```python
from build123d import *

# Parameters (mm, degrees)
CUT_EXTRUDE1_REACH = 6
SKETCH3_R          = 1.5875


with BuildPart() as part:
    # Sketch2 → Revolve1 (revolve)
    with BuildSketch(Plane.XY):
        Polygon((-16, -4), (0, -4), (0, -16.000000004), (-4, -16.000000004), (-4, -8), (-16, -8), align=None)
    revolve(axis=Axis((-12.310421286, 0, 0), (1, 0, 0)))

    # Sketch3 → Cut-Extrude1 (cut, up to next)
    with BuildSketch(Plane.ZY.offset(4), mode=Mode.PRIVATE) as cut_extrude1_sk1:
        with Locations((-9.525, 9.525)):
            Circle(SKETCH3_R)
    cut_extrude1_tool1 = extrude(cut_extrude1_sk1.sketch, amount=-CUT_EXTRUDE1_REACH, mode=Mode.PRIVATE) & part.part
    add(cut_extrude1_tool1.solids().sort_by_distance((-4, 9.525, -9.525))[0], mode=Mode.SUBTRACT)
    # Sketch3 → Cut-Extrude1 (cut, up to next)
    with BuildSketch(Plane.ZY.offset(4), mode=Mode.PRIVATE) as cut_extrude1_sk2:
        with Locations((-9.525, -9.525)):
            Circle(SKETCH3_R)
    cut_extrude1_tool2 = extrude(cut_extrude1_sk2.sketch, amount=-CUT_EXTRUDE1_REACH, mode=Mode.PRIVATE) & part.part
    add(cut_extrude1_tool2.solids().sort_by_distance((-4, -9.525, -9.525))[0], mode=Mode.SUBTRACT)
    # Sketch3 → Cut-Extrude1 (cut, up to next)
    with BuildSketch(Plane.ZY.offset(4), mode=Mode.PRIVATE) as cut_extrude1_sk3:
        with Locations((9.525, -9.525)):
            Circle(SKETCH3_R)
    cut_extrude1_tool3 = extrude(cut_extrude1_sk3.sketch, amount=-CUT_EXTRUDE1_REACH, mode=Mode.PRIVATE) & part.part
    add(cut_extrude1_tool3.solids().sort_by_distance((-4, -9.525, 9.525))[0], mode=Mode.SUBTRACT)
    # Sketch3 → Cut-Extrude1 (cut, up to next)
    with BuildSketch(Plane.ZY.offset(4), mode=Mode.PRIVATE) as cut_extrude1_sk4:
        with Locations((9.525, 9.525)):
            Circle(SKETCH3_R)
    cut_extrude1_tool4 = extrude(cut_extrude1_sk4.sketch, amount=-CUT_EXTRUDE1_REACH, mode=Mode.PRIVATE) & part.part
    add(cut_extrude1_tool4.solids().sort_by_distance((-4, 9.525, 9.525))[0], mode=Mode.SUBTRACT)


solid = part.part
```
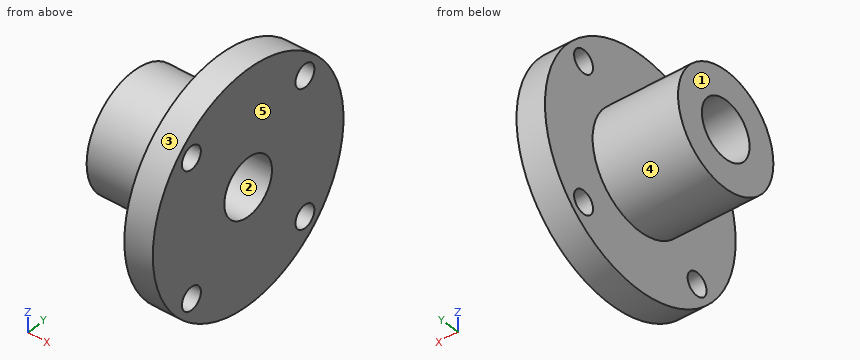
Geometry check sheet. Reference: the model listing, model coordinates, mm. Face numbers are marked on the shaded views. A direction names the side the tool comes from. Round coordinates to 2 decimals unless told otherwise and drop trailing zeros. Write each loop counter-clockwise with the first axis right and the second up, starting at its lowest first coordinate (ties: lowest second). Pieces come first, ordered by that corner, then holes. Notation, with made-up numbers: (10, 79) - (28, 79) arc R30 ccw to (28, 118) - close; hole circle Ø4 at (76.25, 10.25). An arc over 180 degrees is marked (long way). Write each question's results on one line, items separated by ' | '.
(1) Sectioned sample at A-A, the plane y = 0. Enter the section's corners in (x, z).
Computed:
outline: (-16, -8) - (-4, -8) - (-4, -16) - (0, -16) - (0, -4) - (-16, -4) - close; (-16, 4) - (0, 4) - (0, 16) - (-4, 16) - (-4, 8) - (-16, 8) - close
(2) Sectioned sample at C-C, the plane x = -3.25. Enter the section's corners in (y, z) (1 decimal).
Computed:
outline: circle Ø32 at (0, 0); hole circle Ø3.2 at (-9.5, -9.5); hole circle Ø3.2 at (-9.5, 9.5); hole circle Ø8 at (0, 0); hole circle Ø3.2 at (9.5, -9.5); hole circle Ø3.2 at (9.5, 9.5)
(3) Set-up check for the marked faces 4 and 5: record each of +Z, -Z, +X, -X, +Y, -Y from which the full face is reachable in a straight line by a thin tool's end or side.
Computed:
face 4: -X | face 5: +Z, -Z, +X, +Y, -Y
(4) Thickness scan on probe 1 along Z at (x, y) = (-6.5, 0); probe 2 along X at (y, z) = (5, -12); probe 3 along Z at (x, y) = (-3.25, -1.5). Record the ranges inside material, lowest first. Write a range as from..to.
Computed:
probe 1: z = -8..-4, 4..8 | probe 2: x = -4..0 | probe 3: z = -15.93..-3.71, 3.71..15.93
(5) Draft check along Y on the marked faces 1, 2 and 3. Enter one of: pulls with the +Y half, pulls with the -Y half, needs draft (parallel to the pull), parting line crosses it, or undercut.
Computed:
face 1: needs draft | face 2: undercut | face 3: parting line crosses it
(6) Depth check by flat-ended pin: pin 1 Ø8 at (x, y) = (-7, 2.5) entering from +Z; pin 2 Ø3.5 at (y, z) = (-9.525, -9.525) entering from -X; pin 3 Ø2 at (x, y) = (-5.5, 7) entering from +Z; pin 4 Ø2 at (x, z) = (-13.5, -1.5) entering from -Y. Enter the tip coordinate at first touch or a pass-through.
Computed:
pin 1: stops at z = 16 | pin 2: stops at x = -4 | pin 3: stops at z = 5.29 | pin 4: stops at y = -7.98
(7) Sectioned sample at D-D, the plane z = -4.5. Enter the section's corners in (x, y).
Computed:
outline: (-16, -6.61) - (-4, -6.61) - (-4, -15.35) - (0, -15.35) - (0, 15.35) - (-4, 15.35) - (-4, 6.61) - (-16, 6.61) - close
